Can you work these out from the model? Positions are in its coordinate system, mm. A direction names the side the tool comes from. Coordinates: 2 decimals unless noted, no trailing zeros. Order: outer loops, then holes, each group sorted by start corner. A loop starts at its lowest first (then second) coordinate and runs counter-clockwise, first axis right, second up. Notation, with made-up numbers: (3.25, -34.75) -> (37.25, -34.75) arc R17 ccw to (37.25, -25.75) -> close; hole circle Ø9 at (86.25, 29.5). An arc over 180 degrees is marked (long way). Return JSON: item names as keys, results as strings. Group by question number.
1) Thinking about a two-plate mould opening in Y: for faces 4 (the flat face through (-70, 1, 30)), 5 (the flat face through (-120, 15, 57)), 6 (the flat face through (-68, 13, 59)), which applies, +Y half, -Y half, draft (parallel to the pull), parting line (faces both ways), or undercut?
2) For pin 1 (3 mm diameter, centred on x = -70, y = 12, fed in from +Z); pin 2 (1 mm diameter, centred on x = -130.5, y = 15, fed in from -Z); pin 3 (22.5 mm diameter, centred on x = -65.5, z = -29, fed in from +Y), each with a flat end and sliding along its axis, tell me the tip position at first contact or that it passes through.
3) If I drill on probe 1 along Y at (x, z) = (-160, -16); probe 2 along Z at (x, y) = (-109.5, 19), over which ranges is the centre line in solid material (lowest first)? Write a range as from..to.
4) If we section it at A-A, the plane y = 16.5: Please give me the cut outline in (x, z).
5) If we section it at B-B, the plane z = 34: Please give me the cut outline in (x, y), then the cut area to 3 significant figures.
6) If we section it at C-C, the plane z = -47: Please give me the cut outline in (x, y).
7) For faces 1 (the flat face through (-119, 25, 59)), 2 (the flat face through (-70, 1, -30)), 3 (the flat face through (-119, 2, -3)), which set-ups out of +Z, -Z, +X, -X, +Y, -Y let a thin tool reach every point of the face, with its end or its side?
Autodesk Inventor part; units mm, degrees
ref_plane "YZ Plane" through (0, 0, 0) normal (1, 0, 0) x (0, 1, 0)
ref_plane "XZ Plane" through (0, 0, 0) normal (0, 1, 0) x (-1, 0, 0)
ref_plane "XY Plane" through (0, 0, 0) normal (0, 0, 1) x (1, 0, 0)
sketch "スケッチ1" plane through (0, 0, 0) normal (0, 1, 0) x (-1, 0, 0)
  line L0 (180, 60) -> (-180, 60)
  line L1 (-180, 60) -> (-180, -60)
  line L2 (-180, -60) -> (180, -60)
  line L3 (180, -60) -> (180, 60)
  line L4 (180, 60) -> (-180, -60) construction
  line L5 (-180, 60) -> (180, -60) construction
  line L6 (180, 57) -> (-180, 57)
  line L7 (-60, 60) -> (-60, -60)
  line L8 (-60, 40) -> (-80, 40)
  line L9 (-80, 40) -> (-80, 20)
  line L10 (-80, 20) -> (-60, 20)
  line L11 (252, 0) -> (-252, 0) construction
  line L12 (-60, -40) -> (-80, -40)
  line L13 (-80, -40) -> (-80, -20)
  line L14 (-80, -20) -> (-60, -20)
  line L15 (0, -84) -> (0, 84) construction
  line L16 (60, 60) -> (60, -60)
  line L17 (60, 40) -> (80, 40)
  line L18 (80, 40) -> (80, 20)
  line L19 (80, 20) -> (60, 20)
  line L20 (60, -40) -> (80, -40)
  line L21 (80, -20) -> (60, -20)
  line L22 (80, -40) -> (80, -20)
  line L23 (-60, 19.7) -> (-80.3, 19.7)
  line L24 (-80.3, 19.7) -> (-80.3, 40.3)
  line L25 (-80.3, 40.3) -> (-60, 40.3)
  line L26 (-60, -19.7) -> (-80.3, -19.7)
  line L27 (-80.3, -19.7) -> (-80.3, -40.3)
  line L28 (-80.3, -40.3) -> (-60, -40.3)
  line L29 (60, 19.7) -> (80.3, 19.7)
  line L30 (80.3, 19.7) -> (80.3, 40.3)
  line L31 (80.3, 40.3) -> (60, 40.3)
  line L32 (60, -19.7) -> (80.3, -19.7)
  line L33 (80.3, -19.7) -> (80.3, -40.3)
  line L34 (80.3, -40.3) -> (60, -40.3)
  point P0 (0, 0)
  point P1 (60, 57)
  dimension "d0" = 120
  dimension "d1" = 360
  dimension "d4" = 3
  dimension "d5" = 120
  dimension "d7" = 20
  dimension "d8" = 20
  dimension "d9" = 20
  dimension "d10" = 0.3
  dimension "d11" = 0.3
extrude "押し出し3" add sketch "スケッチ1" along normal blind 25 contours L3 L6 L16 L0 | L16 L6 L7 L0 | L7 L6 L1 L0
sketch "スケッチ2" plane through (-180, 0, 60) normal (0, 0, 1) x (1, 0, 0)
  line L0 (0, 0) -> (360, 0)
  line L1 (360, 0) -> (360, 25)
  line L2 (0, 25) -> (360, 25)
  line L3 (0, 0) -> (0, 25)
  line L4 (240, 0) -> (240, 25)
  line L5 (240, 7.5) -> (255, 7.5)
  line L6 (255, 7.5) -> (255, 17.5)
  line L7 (255, 17.5) -> (240, 17.5)
  line L8 (180, -5) -> (180, 30) construction
  line L9 (120, 0) -> (120, 25)
  line L10 (120, 7.5) -> (105, 7.5)
  line L11 (105, 7.5) -> (105, 17.5)
  line L12 (105, 17.5) -> (120, 17.5)
  line L13 (240, 17.9) -> (255.4, 17.9)
  line L14 (255.4, 17.9) -> (255.4, 7.1)
  line L15 (255.4, 7.1) -> (240, 7.1)
  line L16 (120, 17.9) -> (104.6, 17.9)
  line L17 (104.6, 17.9) -> (104.6, 7.1)
  line L18 (104.6, 7.1) -> (120, 7.1)
  point P0 (180, 0)
  point P1 (360, 12.5)
  dimension "d16" = 120
  dimension "d17" = 10
  dimension "d18" = 15
  dimension "d19" = 7.5
  dimension "d24" = 0.4
extrude "押し出し6" add sketch "スケッチ1" along normal blind 2 contours L3 L2 L16 L34 L33 L32 L29 L30 L31 L6 | L31 L30 L29 L16 L19 L18 L17 | L17 L18 L19 L16 | L16 L20 L22 L21 L32 L33 L34 | L16 L21 L22 L20
extrude "押し出し7" cut sketch "スケッチ2" along normal up to surface (3 mm away) from surface at -3 contours L9 L2 L4 L0 | L4 L15 L14 L13 L2 L1 L0 | L4 L5 L6 L7 L13 L14 L15 | L4 L7 L6 L5
extrude "押し出し8" cut sketch "スケッチ2" against normal blind 1 contours L18 L17 L16 L9 L12 L11 L10 | L10 L11 L12 L9
extrude "押し出し9" cut sketch "スケッチ1" against normal blind 1 from surface at 2 contours L31 L30 L29 L16 L19 L18 L17 | L17 L18 L19 L16 | L16 L20 L22 L21 L32 L33 L34 | L16 L21 L22 L20
fillet "フィレット3" radius 4 1 edges at (-120, 2, 57)
fillet "フィレット4" radius 1 2 edges at (-180, 15.5, 57) (-180, 2, -3.5)
properties part number "protectar1"
Result sheet:
{
 "1": {"face 4": "+Y half", "face 5": "draft", "face 6": "undercut"},
 "2": {"pin 1": "stops at z = 59", "pin 2": "stops at z = 57", "pin 3": "stops at y = 2"},
 "3": {"probe 1": "y = 0..2", "probe 2": "z = 57..60"},
 "4": {"outline": "(-180, 58) arc R1 ccw to (-179, 57) -> (-60, 57) -> (-60, 59) -> (-75.4, 59) -> (-75.4, 60) -> (-180, 60) -> close"},
 "5": {"outline": "(-180, 0) -> (-60, 0) -> (-60, 1) -> (-80.3, 1) -> (-80.3, 2) -> (-179, 2) arc R1 ccw to (-180, 1) -> close", "area": "219 mm2"},
 "6": {"outline": "(-180, 0) -> (-60, 0) -> (-60, 2) -> (-179, 2) arc R1 ccw to (-180, 1) -> close"},
 "7": {"face 1": "+Z, -Z, +X, -X, +Y", "face 2": "+X, +Y", "face 3": "-Z, +X, -X, +Y"}
}
